Geometry: see drawing. Coordinates: mm, zero at the bounding-box minimum. Give positions to 0.01 mm unless a question says otherwise; leave off trailing zeros. Write each loop counter-clockwise with the first axis right and the second up, starting at its lowest first coordinate (ties: lowest second). Pieces come first, ordered by that corner, then holes.
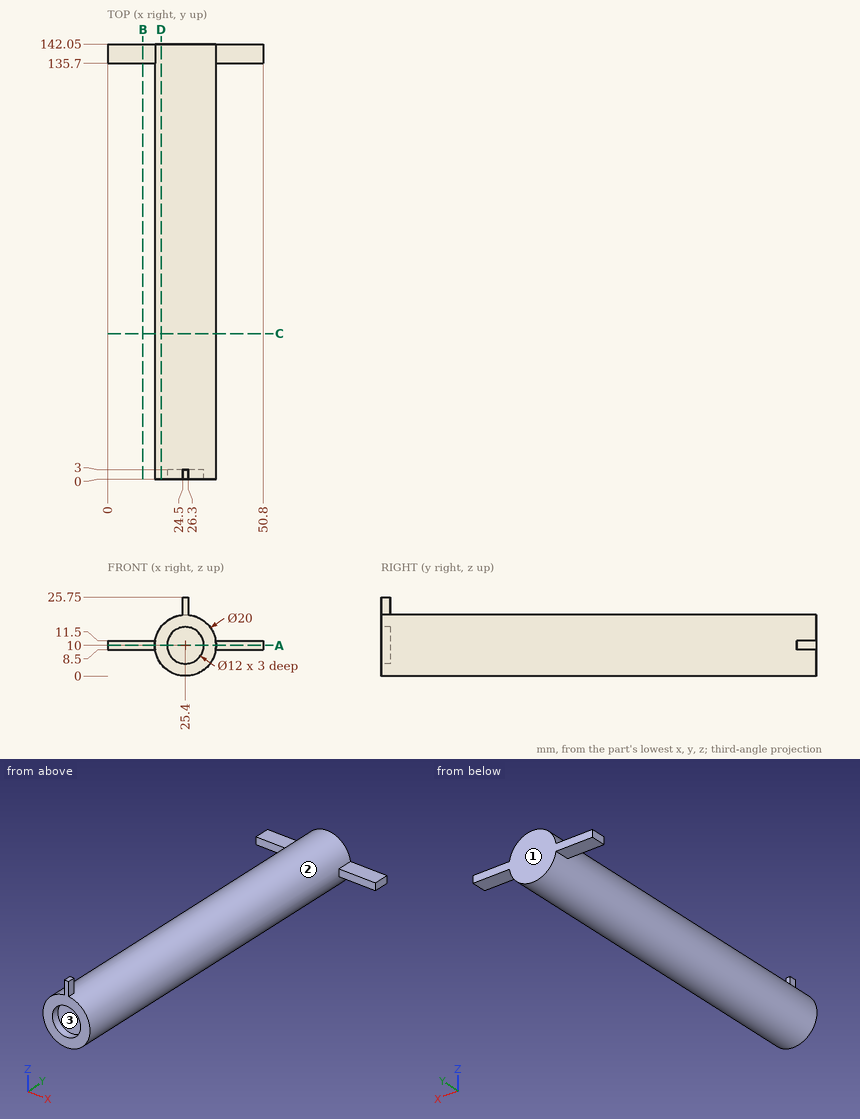
1. Line query: probe 1 along Z at (x, y) = (25.4, 1.45); probe 2 along X at (y, z) = (67.5, 8.5); probe 3 along Y at (x, z) = (20.5, 7.25). Output: solid intervals per line, ascending.
2. Section query B-B (x = 11.5). Return loops of the section in (y, z), plus the area to 4 significant figures.
3. Pin query (flat end, axial travel): P1, Ø8, axis at x = 22, y = 82, coming from the +Z side; P2, Ø3, axis at x = 7.5, y = 137.5, coming from the +Z side; P3, Ø5, axis at y = 67.5, z = 11.5, coming from the -X side. Return the tip coordinate at first contact, or that it passes through.
4. Section query A-A (z = 10). Return loops of the section in (x, y), plus the area to 3 significant figures.
5. Section query C-C (y = 47.5). Return loops of the section in (x, z), plus the area to 3 significant figures.
6. Pull-direction query (X, two-part tool) for the marked faces 1, 2 and 3; classes: pulls with the +X half, pulls with the -X half, needs draft (parallel to the pull), parting line crosses it, or undercut.
7. Section query D-D (x = 17.5). Return loops of the section in (y, z), plus the area to 3 significant figures.
The answers:
1. probe 1: z = 0 to 4, 16 to 25.75
1. probe 2: x = 15.51 to 35.29
1. probe 3: y = 3 to 142.05
2. outline: (135.7, 8.5) - (142.05, 8.5) - (142.05, 11.5) - (135.7, 11.5) - close
2. area: 19.05 mm2
3. P1: stops at z = 20
3. P2: stops at z = 11.5
3. P3: stops at x = 15.4
4. outline: (0, 135.7) - (15.4, 135.7) - (15.4, 0) - (19.4, 0) - (19.4, 3) - (31.4, 3) - (31.4, 0) - (35.4, 0) - (35.4, 135.7) - (50.8, 135.7) - (50.8, 142.05) - (0, 142.05) - close
4. area: 3,000 mm2
5. outline: circle Ø20 at (25.4, 10)
5. area: 314 mm2
6. face 1: needs draft
6. face 2: parting line crosses it
6. face 3: undercut
7. outline: (0, 3.87) - (142.05, 3.87) - (142.05, 16.13) - (0, 16.13) - close
7. area: 1,740 mm2
